```python
from build123d import *

# Parameters (mm, degrees)
SALIENTE_EXTRUIR1_DEPTH = 12.7
CROQUIS2_R              = 20
CORTAR_EXTRUIR1_DEPTH   = 12.7
CROQUIS4_R              = 3
CORTAR_EXTRUIR3_DEPTH   = 3
CROQUIS5_R              = 35
CORTAR_EXTRUIR4_DEPTH   = 4
CROQUIS6_R              = 1.5
CORTAR_EXTRUIR5_DEPTH   = 22
CROQUIS7_R              = 35
CORTAR_EXTRUIR6_DEPTH   = 10
CORTAR_EXTRUIR6_DRAFT   = -45
CROQUIS8_R              = 1.5
CORTAR_EXTRUIR7_DEPTH   = 29
CROQUIS9_R              = 2.5
CORTAR_EXTRUIR8_DEPTH   = 20
CROQUIS10_R             = 2.5
CORTAR_EXTRUIR9_DEPTH   = 20


with BuildPart() as part:
    # Croquis1 → Saliente-Extruir1 (new body)
    with BuildSketch(Plane.XY):
        with BuildLine():
            Line((-106.743982658, 74.697593063), (43.256017342, 74.697593063))
            ThreePointArc((43.256017342, 74.697593063), (50.327085153, 71.768660875), (53.256017342, 64.697593063))
            Line((53.256017342, 64.697593063), (53.256017342, 40.697593063))
            Line((53.256017342, 40.697593063), (53.256017342, -39.302406937))
            ThreePointArc((53.256017342, -39.302406937), (50.327085153, -46.373474748), (43.256017342, -49.302406937))
            Line((43.256017342, -49.302406937), (-46.743982658, -49.302406937))
            Line((-46.743982658, -49.302406937), (-77.581038689, -49.302406937))
            ThreePointArc((-77.581038689, -49.302406937), (-84.60035231, -46.424852885), (-87.579975061, -39.448254194))
            ThreePointArc((-87.579975061, -39.448254194), (-93.601441457, -23.536626284), (-108.410649325, -15.162539908))
            ThreePointArc((-108.410649325, -15.162539908), (-114.381608817, -11.75737918), (-116.743982658, -5.302406937))
            Line((-116.743982658, -5.302406937), (-116.743982658, 64.697593063))
            ThreePointArc((-116.743982658, 64.697593063), (-113.81505047, 71.768660875), (-106.743982658, 74.697593063))
        make_face()
    extrude(amount=SALIENTE_EXTRUIR1_DEPTH)

    # Croquis2 → Cortar-Extruir1 (cut)
    with BuildSketch(Plane(origin=(0, 0, 0), x_dir=(-1, 0, 0), z_dir=(0, 0, -1))):
        with Locations((-3.256017342, 10.697593063)):
            Circle(CROQUIS2_R)
    extrude(amount=-CORTAR_EXTRUIR1_DEPTH, mode=Mode.SUBTRACT)

    # Croquis4 → Cortar-Extruir3 (cut)
    with BuildSketch(Plane(origin=(0, 0, 0), x_dir=(-1, 0, 0), z_dir=(0, 0, -1))):
        with Locations((36.743982658, 48.697593063)):
            Circle(CROQUIS4_R)
        with Locations((-43.256017342, 48.697593063)):
            Circle(CROQUIS4_R)
        with Locations((36.743982658, -31.302406937)):
            Circle(CROQUIS4_R)
        with Locations((-43.256017342, -31.302406937)):
            Circle(CROQUIS4_R)
    extrude(amount=-CORTAR_EXTRUIR3_DEPTH, mode=Mode.SUBTRACT)

    # Croquis5 → Cortar-Extruir4 (cut)
    with BuildSketch(Plane(origin=(0, 0, 0), x_dir=(-1, 0, 0), z_dir=(0, 0, -1))):
        with Locations((-3.256017342, 10.697593063)):
            Circle(CROQUIS5_R)
    extrude(amount=-CORTAR_EXTRUIR4_DEPTH, mode=Mode.SUBTRACT)

    # Croquis6 → Cortar-Extruir5 (cut)
    with BuildSketch(Plane(origin=(0, 0, 4), x_dir=(-1, 0, 0), z_dir=(0, 0, -1))):
        with Locations((-3.256017342, 42.697593063)):
            Circle(CROQUIS6_R)
        with Locations((19.371399656, 33.325010061)):
            Circle(CROQUIS6_R)
        with Locations((28.743982658, 10.697593063)):
            Circle(CROQUIS6_R)
        with Locations((19.371399656, -11.929823935)):
            Circle(CROQUIS6_R)
        with Locations((-3.256017342, -21.302406937)):
            Circle(CROQUIS6_R)
        with Locations((-25.88343434, -11.929823935)):
            Circle(CROQUIS6_R)
        with Locations((-35.256017342, 10.697593063)):
            Circle(CROQUIS6_R)
        with Locations((-25.88343434, 33.325010061)):
            Circle(CROQUIS6_R)
    extrude(amount=-CORTAR_EXTRUIR5_DEPTH, mode=Mode.SUBTRACT)


with BuildPart() as cortar_extruir6_tool:
    # Croquis7 → Cortar-Extruir6 (with draft: the straight prism first)
    with BuildSketch(Plane(origin=(0, 0, 4), x_dir=(-1, 0, 0), z_dir=(0, 0, -1))):
        with Locations((-3.256017342, 10.697593063)):
            Circle(CROQUIS7_R)
    extrude(amount=CORTAR_EXTRUIR6_DEPTH)
    # Cortar-Extruir6: the draft: its side faces are tilted about the plane it starts from
    cortar_extruir6_sides = [cortar_extruir6_tool.faces().sort_by_distance(p)[0] for p in [
        (38.256017342, 10.697593063, -1),
    ]]
    draft(cortar_extruir6_sides, Plane(origin=(0, 0, 4), x_dir=(-1, 0, 0), z_dir=(0, 0, -1)), CORTAR_EXTRUIR6_DRAFT)


with BuildPart() as part_1:
    add(part.part)

    # Cortar-Extruir6: cut by cortar_extruir6_tool
    add(cortar_extruir6_tool.part, mode=Mode.SUBTRACT)

    # Croquis8 → Cortar-Extruir7 (cut)
    with BuildSketch(Plane(origin=(0, 0, 0), x_dir=(-1, 0, 0), z_dir=(0, 0, -1))):
        with Locations((-43.256017342, 48.697593063)):
            Circle(CROQUIS8_R)
        with Locations((36.743982658, 48.697593063)):
            Circle(CROQUIS8_R)
        with Locations((36.743982658, -31.302406937)):
            Circle(CROQUIS8_R)
        with Locations((-43.256017342, -31.302406937)):
            Circle(CROQUIS8_R)
    extrude(amount=-CORTAR_EXTRUIR7_DEPTH, mode=Mode.SUBTRACT)

    # Croquis9 → Cortar-Extruir8 (cut)
    with BuildSketch(Plane(origin=(0, 74.697593063, 0), x_dir=(1, 0, 0), z_dir=(0, 1, 0))):
        with Locations(Location((-91.743982658, -6.35, 0), (0, 0, 270))):
            Circle(CROQUIS9_R)
        with Locations(Location((-71.743982658, -6.35, 0), (0, 0, 270))):
            Circle(CROQUIS9_R)
        with Locations(Location((-51.743982658, -6.35, 0), (0, 0, 270))):
            Circle(CROQUIS9_R)
    extrude(amount=-CORTAR_EXTRUIR8_DEPTH, mode=Mode.SUBTRACT)

    # Croquis10 → Cortar-Extruir9 (cut)
    with BuildSketch(Plane.ZY.offset(116.743982658)):
        with Locations((6.35, 49.697593063)):
            Circle(CROQUIS10_R)
        with Locations((6.35, 29.697593063)):
            Circle(CROQUIS10_R)
        with Locations((6.35, 9.697593063)):
            Circle(CROQUIS10_R)
    extrude(amount=-CORTAR_EXTRUIR9_DEPTH, mode=Mode.SUBTRACT)


solid = part_1.part
```
Check sheet for the modelled part. Datum: model origin and axes. Units: mm. A direction names the side the tool comes from. Give positions to 0.01 mm unless a question says otherwise; leave off trailing zeros. Order: outer loops, then holes, each group sorted by start corner. A loop starts at its lowest first (then second) coordinate and runs counter-clockwise, first axis right, second up. Notation, with made-up numbers: (54.5, -17.5) -> (95.5, -17.5) arc R24 cw to (95.5, -4.5) -> close; hole circle Ø4 at (-28, 17.25). An arc over 180 degrees is marked (long way). Return JSON: item names as keys, results as strings.
1. Cross-section at B-B, the plane z = 6.35. Count the separate pieces of the cut face and the enclosed holes in it, plus the area to 3 significant figures.
From the geometry:
{"separate pieces": "1", "enclosed holes": "13", "area": "18,200 mm^2"}
2. Mould release check, pull along Z, two halves, no side actions. Record for faces 1 (the cylindrical face through (-94.185, 64.838, 5.808)), 2 (the cylindrical face through (-106.884, 32.176, 6.025)), 3 (the cylindrical face through (50.249, 71.846, 6.261)), 4 (the conical face through (-30.31, 21.27, 3.81)): +Z half, -Z half, draft (parallel to the pull), parting line (faces both ways), or undercut.
From the geometry:
{"face 1": "undercut", "face 2": "undercut", "face 3": "draft", "face 4": "-Z half"}
3. Go/stop test with flat-tipped pins: P1, Ø5, axis at y = -27, z = 5.5, coming from the -X side; P2, Ø5, axis at x = 25.88, y = -11.93, coming from the -Z side; P3, Ø5, axis at y = -34.5, z = 7.5, coming from the -X side; P4, Ø2.5, axis at x = 3.26, y = 42.7, coming from the +Z side. Record where each tip stops, or that it passes through.
From the geometry:
{"P1": "x = -92.82", "P2": "z = 4", "P3": "x = -88.83", "P4": "through"}
4. Material ranges on probe 1 along X at (y, z) = (42.5, 10.25); probe 2 along X at (y, z) = (55.5, 5.75); probe 3 along X at (y, z) = (-3.5, 6), recorded low to high. Write a range as [from, to].
From the geometry:
{"probe 1": "[-116.74, 1.77], [4.74, 53.26]", "probe 2": "[-116.74, -94.17], [-89.32, -74.17], [-69.32, -54.17], [-49.32, 53.26]", "probe 3": "[-116.74, -10.83], [17.34, 53.26]"}
5. Set-up check for faces 5 (the cylindrical face through (-106.884, 8.176, 4.366)), 6 (the cylindrical face through (-74.185, 64.838, 5.808)), 7 (the flat face through (-35, -32, 3)): record each of +Z, -Z, +X, -X, +Y, -Y from which the full face is reachable in a straight line by a thin tool's end or side.
From the geometry:
{"face 5": "-X", "face 6": "+Y", "face 7": "-Z"}
6. Cross-section at A-A, the plane x = -99.5. Record the cut outline in (y, z), plus the area to 3 significant figures.
From the geometry:
{"outline": "(-18.51, 0) -> (74.7, 0) -> (74.7, 12.7) -> (-18.51, 12.7) -> close; hole circle Ø5 at (9.7, 6.35); hole circle Ø5 at (29.7, 6.35); hole circle Ø5 at (49.7, 6.35)", "area": "1,120 mm^2"}
